Autodesk Inventor part; units mm, degrees
ref_plane "YZ Plane" through (0, 0, 0) normal (1, 0, 0) x (0, 1, 0)
ref_plane "XZ Plane" through (0, 0, 0) normal (0, 1, 0) x (-1, 0, 0)
ref_plane "XY Plane" through (0, 0, 0) normal (0, 0, 1) x (1, 0, 0)
sketch "Sketch1" plane through (0, 0, 0) normal (0, 1, 0) x (-1, 0, 0)
  line L0 (-9.398, 3.81) -> (9.398, 3.81)
  line L1 (9.398, 3.81) -> (9.398, -3.81)
  line L2 (9.398, -3.81) -> (-9.398, -3.81)
  line L3 (-9.398, -3.81) -> (-9.398, 3.81)
  line L4 (-9.398, 3.81) -> (9.398, -3.81) construction
  line L5 (9.398, 3.81) -> (-9.398, -3.81) construction
  point P0 (0, 0)
  dimension "d0" = 18.796
  dimension "d1" = 7.62
extrude "Extrusion1" add sketch "Sketch1" along normal blind 3.175
sketch "Sketch2" plane through (0, 3.175, 0) normal (0, 1, 0) x (1, 0, 0)
  line L0 (-9.398, -3.81) -> (9.398, -3.81)
  line L1 (3.683, 3.81) -> (-3.683, 3.81)
  line L2 (-3.683, 3.81) -> (-3.683, -3.81)
  line L3 (-3.683, -3.81) -> (3.683, -3.81)
  line L4 (3.683, -3.81) -> (3.683, 3.81)
  line L5 (3.683, 3.81) -> (-3.683, -3.81) construction
  line L6 (-3.683, 3.81) -> (3.683, -3.81) construction
  point P0 (0, 0)
  dimension "d4" = 7.366
extrude "Extrusion2" add sketch "Sketch2" along normal blind 4.445
sketch "Sketch3" plane through (0, 7.62, 0) normal (0, 1, 0) x (1, 0, 0)
  circle A0 centre (0, 0) radius 3.7
  dimension "d7" = 7.4
extrude "Extrusion3" add sketch "Sketch3" along normal blind 34
properties part number "Press_Mandrel"
Here's how the part is built. I have some questions about the finished solid (model axes, mm). A direction names the side the tool comes from. Give positions to 0.01 mm unless a question says otherwise; leave off trailing zeros. Order: outer loops, then holes, each group sorted by start corner. A loop starts at its lowest first (then second) coordinate and runs counter-clockwise, first axis right, second up. Notation, with made-up numbers: M 77,-0.75 L 130,-0.75 A23 cw 130,13.25 Z; hole C 73.25,21.5 d3. An arc over 180 degrees is marked long. Answer as a JSON object with one key per item and string values. Group by question number.
1) Suppose I cut it at C-C, the plane y = 20. Write out the boundary of the cut face in (x, z).
2) Please list where these lines run through material, in increasing order: L1, parallel to X at y = 15, z = -0.25; L2, parallel to Y at x = 4, z = 0 (3 decimals); L3, parallel to X at y = 28, z = -3. Write a range as [from, to].
3) Suppose I cut it at D-D, the plane z = 2.5. Write out the boundary of the cut face in (x, y) (3 decimals).
4) Suppose I cut it at A-A, the plane x = 0. Write out the boundary of the cut face in (y, z), plus the area to 3 significant figures.
5) Suppose I cut it at B-B, the plane z = -3. Write out the boundary of the cut face in (x, y) (3 decimals), plus the area to 3 significant figures.
6) I'm going to push flat-ended pins straight in: pin 1 Ø4.5 at (x, z) = (-7.5, -1.5) entering from +Y (3 decimals); pin 2 Ø3 at (y, z) = (33.5, -2.5) entering from +X; pin 3 Ø3 at (y, z) = (30, 1.5) entering from +X. Where does each tip first touch, or does it pass through?
7) On a 3-axis mill with a long thin cutter (end or side, diameter ignored), from which of +Z, -Z, +X, -X, +Y, -Y can I reach the whole of each face in a straight line? I mean faces 1 (the cylindrical face through (-0.802, 24.382, -3.612)), 2 (the flat face through (0, 3, -3.81)). Say none if no direction works.
Results found:
{
 "1": {"outline": "C 0,0 d7.4"},
 "2": {"L1": "[-3.69, 3.69]", "L2": "[0, 3.175]", "L3": "[-2.17, 2.17]"},
 "3": {"outline": "M -9.398,0 L 9.398,0 L 9.398,3.175 L 3.683,3.175 L 3.683,7.62 L 2.728,7.62 L 2.728,41.62 L -2.728,41.62 L -2.728,7.62 L -3.683,7.62 L -3.683,3.175 L -9.398,3.175 Z"},
 "4": {"outline": "M 0,-3.81 L 7.62,-3.81 L 7.62,-3.7 L 41.62,-3.7 L 41.62,3.7 L 7.62,3.7 L 7.62,3.81 L 0,3.81 Z", "area": "310 mm²"},
 "5": {"outline": "M -9.398,0 L 9.398,0 L 9.398,3.175 L 3.683,3.175 L 3.683,7.62 L 2.166,7.62 L 2.166,41.62 L -2.166,41.62 L -2.166,7.62 L -3.683,7.62 L -3.683,3.175 L -9.398,3.175 Z", "area": "240 mm²"},
 "6": {"pin 1": "y = 3.175", "pin 2": "x = 3.56", "pin 3": "x = 3.7"},
 "7": {"face 1": "+Y", "face 2": "-Z, +X, -X, +Y, -Y"}
}
